```python
from build123d import *

# Parameters (mm, degrees)
SKETCH1_W           = 80
SKETCH1_H           = 80
BOSS_EXTRUDE1_DEPTH = 2
SKETCH3_R           = 12.5
CUT_EXTRUDE2_DEPTH  = 114.154761279
SKETCH5_R           = 1.5
CUT_EXTRUDE3_DEPTH  = 114.154761279
FILLET1_RADIUS      = 40
FILLET1_LENGTH      = 2


with BuildPart() as part:
    # Sketch1 → Boss-Extrude1 (new body)
    with BuildSketch(Plane(origin=(0, 0, 0), x_dir=(1, 0, 0), z_dir=(0, 1, 0))):
        with Locations((40, 40)):
            Rectangle(SKETCH1_W, SKETCH1_H)
    extrude(amount=BOSS_EXTRUDE1_DEPTH)

    # Sketch3 → Cut-Extrude2 (cut, through all)
    with BuildSketch(Plane(origin=(0, 2, 0), x_dir=(1, 0, 0), z_dir=(0, 1, 0))):
        with Locations(Location((40, 40, 0), (0, 0, 270))):
            Circle(SKETCH3_R)
    extrude(amount=-CUT_EXTRUDE2_DEPTH, mode=Mode.SUBTRACT)

    # Sketch5 → Cut-Extrude3 (cut, through all)
    with BuildSketch(Plane(origin=(0, 2, 0), x_dir=(1, 0, 0), z_dir=(0, 1, 0))):
        with Locations(Location((22.68, 30.000293338, 0), (0, 0, 270))):
            Circle(SKETCH5_R)
        with Locations(Location((57.32, 30.000293338, 0), (0, 0, 270))):
            Circle(SKETCH5_R)
        with Locations(Location((40, 59.999413325, 0), (0, 0, 270))):
            Circle(SKETCH5_R)
    extrude(amount=-CUT_EXTRUDE3_DEPTH, mode=Mode.SUBTRACT)

    # Fillet1: full round fillet: the end face becomes a half cylinder, R = half its width
    fillet1_face = Plane((40, 1, -80), x_dir=(0, 1, 0), z_dir=(0, 0, -1))  # on the end face: x along it, z out of the body
    fillet1_slab = fillet1_face.offset(-FILLET1_RADIUS / 2) * Box(FILLET1_LENGTH, 2 * FILLET1_RADIUS, FILLET1_RADIUS, mode=Mode.PRIVATE)  # the body's end, R deep
    fillet1_round = Plane((40, 1, -40), x_dir=(0, 0, -1), z_dir=(0, 1, 0)) * Cylinder(FILLET1_RADIUS, FILLET1_LENGTH, mode=Mode.PRIVATE)  # its axis R under the face
    add(fillet1_slab - fillet1_round, mode=Mode.SUBTRACT)


solid = part.part
```
Design review of the part built by this model. Coordinates are the model's own, in mm. Coordinates: 2 decimals unless noted, no trailing zeros. Write each loop counter-clockwise with the first axis right and the second up, starting at its lowest first coordinate (ties: lowest second). Pieces come first, ordered by that corner, then holes.
1) Add section D-D (x = 22.68). Write out the cut boundary in (y, z), plus the area to 3 significant figures.
2) To check wall thickness, follow L1, parallel to X at y = 1.3, z = -40; L2, parallel to X at y = 0.7, z = -50; L3, parallel to Z at x = 50, y = 1.5. State the ranges of each line that lie inside material, in increasing order.
3) Add section C-C (z = -49). Write out the cut boundary in (x, y), plus the area to 3 significant figures.
4) Add section A-A (x = 40). Write out the cut boundary in (y, z).
5) Add section B-B (y = 0.6). Write out the cut boundary in (x, z).
6) Mouldability with a two-part tool opening along X and no side actions: class faces 1 (the cylindrical face through (39.1, 1, -61.2)), 2 (the cylindrical face through (56.407, 1.014, -31.191)), 3 (the flat face through (0, 1, -20)), 4 (the flat face through (39, 0, -23)) as +X half, -X half, draft (parallel to the pull), parting line (faces both ways), or undercut.
7) Insertion check: pin 1 (1.8 mm diameter, centred on x = 40, z = -60, fed in from +Y). The pin has a flat end and moves straight along its axis. Give the tip position at first contact, or say it passes through.
Check result:
1. outline: (0, -76.06) - (2, -76.06) - (2, -31.5) - (0, -31.5) - close; (0, -28.5) - (2, -28.5) - (2, 0) - (0, 0) - close
1. area: 146 mm2
2. L1: x = 0 to 27.5, 52.5 to 80
2. L2: x = 1.27 to 32.5, 47.5 to 78.73
2. L3: z = -78.73 to -47.5, -32.5 to 0
3. outline: (1.03, 0) - (31.33, 0) - (31.33, 2) - (1.03, 2) - close; (48.67, 0) - (78.97, 0) - (78.97, 2) - (48.67, 2) - close
3. area: 121 mm2
4. outline: (0, -80) - (2, -80) - (2, -61.5) - (0, -61.5) - close; (0, -58.5) - (2, -58.5) - (2, -52.5) - (0, -52.5) - close; (0, -27.5) - (2, -27.5) - (2, 0) - (0, 0) - close
5. outline: (0, -40) arc R40 ccw to (80, -40) - (80, 0) - (0, 0) - close; hole circle Ø3 at (22.68, -30); hole circle Ø25 at (40, -40); hole circle Ø3 at (40, -60); hole circle Ø3 at (57.32, -30)
6. face 1: undercut
6. face 2: undercut
6. face 3: -X half
6. face 4: draft
7. pin 1: passes through
